The model under review builds one solid part; all positions refer to its coordinate system, in mm. Face numbers are marked on the shaded views. Coordinates: 2 decimals unless noted, no trailing zeros. Loops run counter-clockwise (first coordinate to the right, second up) from the corner with the lowest first, then second, coordinate; pieces in that order, holes last. Notation, with made-up numbers: M 89.5,38.5 L 121.5,38.5 A36 cw 121.5,75.5 Z; hole C -32,-25 d7. An arc over 180 degrees is marked long. Return JSON: item names as keys, results as strings.
```python
from build123d import *

# Parameters (mm, degrees)
F0_R     = 7
F1_DEPTH = 4.4
F3_DEPTH = 2.6
F6_R     = 4
F7_DEPTH = 16


with BuildPart() as f1:
    # F0 (on Top) → F1 (new body)
    with BuildSketch(Plane.XY):
        Circle(F0_R)
    extrude(amount=F1_DEPTH)

    # F2 (on face) → F3 (cut)
    with BuildSketch(Plane.XY.offset(4.4)):
        Polygon((2.5, -1.443376), (2.5, 1.443376), (0, 2.886751), (-2.5, 1.443376), (-2.5, -1.443376), (0, -2.886751), align=None)
    extrude(amount=-F3_DEPTH, mode=Mode.SUBTRACT)

    # F4 (on Right) → F5 (revolve, cut)
    with BuildSketch(Plane.YZ):
        with BuildLine():
            Line((-7, 4.4), (-7, 0))
            ThreePointArc((-7, 0), (-6.319513, 2.483371), (-4.6, 4.4))
            Line((-4.6, 4.4), (-7, 4.4))
        make_face()
    revolve(axis=Axis((0, 0, 2.2), (0, 0, 1)), mode=Mode.SUBTRACT)

    # F6 (on Top) → F7 (join)
    with BuildSketch(Plane.XY):
        Circle(F6_R)
    extrude(amount=-F7_DEPTH)


solid = f1.part
```
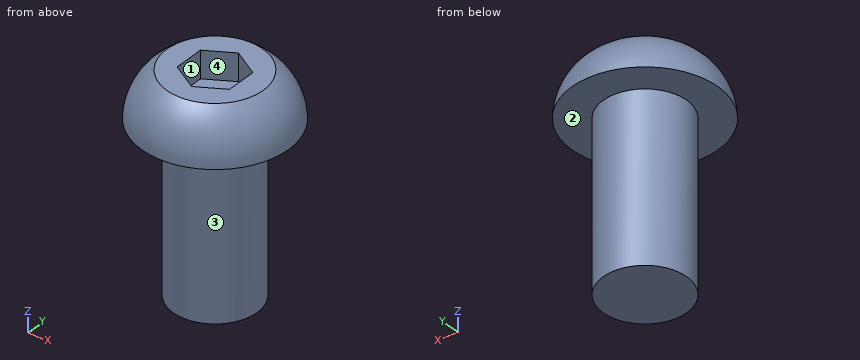
1. The part is to be moulded in two halves that separate along Y. For the marked faces 1, 2, 3 and 4, say which applies: released by +Y, released by -Y, zero draft, split by the parting line, or undercut.
Check values:
{"face 1": "undercut", "face 2": "zero draft", "face 3": "split by the parting line", "face 4": "undercut"}
2. To check wall thickness, follow line 1 (Z direction, x = -2.25, y = 4); line 2 (Z direction, x = -2, y = 1); line 3 (X direction, y = -1, z = -4). State the ranges of each line that lie inside material, in increasing order.
Check values:
{"line 1": "0 to 4.4", "line 2": "-16 to 1.8", "line 3": "-3.87 to 3.87"}
3. Add section A-A on z = -5.5. Give the boundary of the cut face in (x, y), plus the area to 3 significant figures.
Check values:
{"outline": "C 0,0 d8", "area": "50.3 mm²"}
4. Insertion check: pin 1 Ø2 at (y, z) = (0, 2.5) entering from +X; pin 2 Ø6 at (x, z) = (4.5, 1.5) entering from -Y; pin 3 Ø3 at (y, z) = (5, -13) entering from +X. Each pin has a flat end and moves straight along its axis. Give the tip position at first contact, or say it passes through.
Check values:
{"pin 1": "x = 6.74", "pin 2": "y = -6.76", "pin 3": "x = 1.94"}
